For this review, take the finished solid that the model builds, in its own axes (mm). Give positions to 0.01 mm unless a question says otherwise; leave off trailing zeros. Write each loop counter-clockwise with the first axis right and the second up, starting at its lowest first coordinate (ties: lowest second). Pieces come first, ordered by that corner, then holes. Notation, with made-up numbers: (76, 42) -> (92, 42) arc R18 cw to (92, 52) -> close; hole circle Ø7 at (43.25, -0.75). An arc over 180 degrees is marked (long way). Return JSON: item names as keys, results as strings.
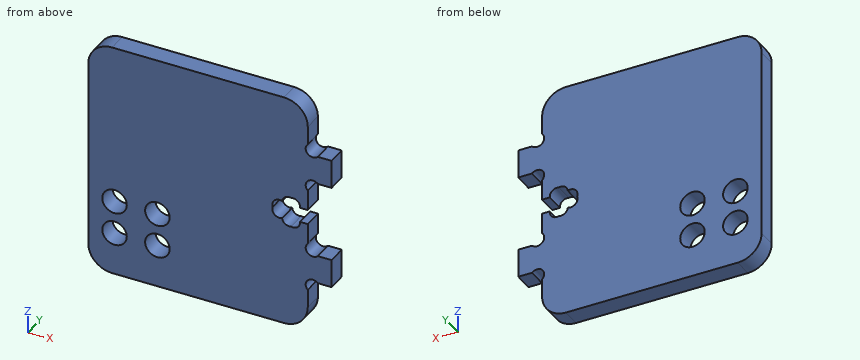
from build123d import *

# Parameters (mm, degrees)
SALIENTE_EXTRUIR1_DEPTH = 4
CORTAR_EXTRUIR4_DEPTH   = 5
CROQUIS10_R             = 1.5
CORTAR_EXTRUIR5_DEPTH   = 5
CROQUIS12_R             = 2.575
CORTAR_EXTRUIR6_DEPTH   = 5


with BuildPart() as part:
    # Croquis1 → Saliente-Extruir1 (new body)
    with BuildSketch(Plane(origin=(0, 0, 0), x_dir=(1, 0, 0), z_dir=(0, 1, 0))):
        with BuildLine():
            Line((-18.025, -25), (18.025, -25))
            ThreePointArc((18.025, -25), (21.560533906, -23.535533906), (23.025, -20))
            Line((23.025, -20), (23.025, -14))
            Line((23.025, -14), (28.025, -14))
            Line((28.025, -14), (28.025, -8))
            Line((28.025, -8), (23.025, -8))
            Line((23.025, -8), (23.025, -1.55))
            Line((23.025, -1.55), (20.975, -1.55))
            Line((20.975, -1.55), (20.975, -2.8))
            Line((20.975, -2.8), (18.075, -2.8))
            Line((18.075, -2.8), (18.075, -1.55))
            Line((18.075, -1.55), (16.025, -1.55))
            Line((16.025, -1.55), (16.025, 1.55))
            Line((16.025, 1.55), (18.075, 1.55))
            Line((18.075, 1.55), (18.075, 2.8))
            Line((18.075, 2.8), (20.975, 2.8))
            Line((20.975, 2.8), (20.975, 1.55))
            Line((20.975, 1.55), (23.025, 1.55))
            Line((23.025, 1.55), (23.025, 8))
            Line((23.025, 8), (28.025, 8))
            Line((28.025, 8), (28.025, 14))
            Line((28.025, 14), (23.025, 14))
            Line((23.025, 14), (23.025, 20))
            ThreePointArc((23.025, 20), (21.560533906, 23.535533906), (18.025, 25))
            Line((18.025, 25), (-18.025, 25))
            ThreePointArc((-18.025, 25), (-21.560533906, 23.535533906), (-23.025, 20))
            Line((-23.025, 20), (-23.025, -20))
            ThreePointArc((-23.025, -20), (-21.560533906, -23.535533906), (-18.025, -25))
        make_face()
    extrude(amount=SALIENTE_EXTRUIR1_DEPTH)

    # Croquis7 → Cortar-Extruir4 (cut, through all)
    with BuildSketch(Plane(origin=(0, 4, 0), x_dir=(1, 0, 0), z_dir=(0, 1, 0))):
        with BuildLine():
            Line((21.402341989, 1.55), (23.025, 1.55))
            Line((23.025, 1.55), (23.025, -1.55))
            Line((23.025, -1.55), (21.402341989, -1.55))
            ThreePointArc((21.402341989, -1.55), (20.900478098, -2.869619136), (19.525, -3.187930349))
            ThreePointArc((19.525, -3.187930349), (18.280747615, -2.971867524), (17.642475162, -1.882163243))
            ThreePointArc((17.642475162, -1.882163243), (16.05076038, -1.575149398), (15.66772275, 0))
            ThreePointArc((15.66772275, 0), (16.05076038, 1.575149398), (17.642475162, 1.882163243))
            ThreePointArc((17.642475162, 1.882163243), (18.280747615, 2.971867524), (19.525, 3.187930349))
            ThreePointArc((19.525, 3.187930349), (20.900478098, 2.869619136), (21.402341989, 1.55))
        make_face()
    extrude(amount=-CORTAR_EXTRUIR4_DEPTH, mode=Mode.SUBTRACT)

    # Croquis10 → Cortar-Extruir5 (cut, through all)
    with BuildSketch(Plane(origin=(0, 4, 0), x_dir=(1, 0, 0), z_dir=(0, 1, 0))):
        with Locations((24.085660172, 15.060660172)):
            Circle(CROQUIS10_R)
        with Locations((24.085660172, 6.939339828)):
            Circle(CROQUIS10_R)
        with Locations((24.085660172, -15.060660172)):
            Circle(CROQUIS10_R)
        with Locations((24.085660172, -6.939339828)):
            Circle(CROQUIS10_R)
    extrude(amount=-CORTAR_EXTRUIR5_DEPTH, mode=Mode.SUBTRACT)

    # Croquis12 → Cortar-Extruir6 (cut, through all)
    with BuildSketch(Plane(origin=(0, 4, 0), x_dir=(1, 0, 0), z_dir=(0, 1, 0))):
        with Locations((-17.525, 16)):
            Circle(CROQUIS12_R)
        with Locations((-8.525, 16)):
            Circle(CROQUIS12_R)
        with Locations((-8.525, 9)):
            Circle(CROQUIS12_R)
        with Locations((-17.525, 9)):
            Circle(CROQUIS12_R)
    extrude(amount=-CORTAR_EXTRUIR6_DEPTH, mode=Mode.SUBTRACT)


solid = part.part
1. To check wall thickness, follow probe 1 along X at (y, z) = (0.35, -16) (3 decimals); probe 2 along Z at (x, y) = (-8, 1.7); probe 3 along Z at (x, y) = (22, 1.6). State the ranges of each line that lie inside material, in increasing order.
Results found:
{"probe 1": "x = -23.025 to -20.1, -14.95 to -11.1, -5.95 to 22.916", "probe 2": "z = -25 to -18.52, -13.48 to -11.52, -6.48 to 25", "probe 3": "z = -23.03 to -1.55, 1.55 to 23.03"}
2. Add section C-C, the plane z = 21.5. State the section outline as (x, y) points.
Results found:
{"outline": "(-22.79, 0) -> (22.79, 0) -> (22.79, 4) -> (-22.79, 4) -> close"}
3. Add section A-A, the plane x = -8.5. State the section outline as (y, z) points, plus the area to 3 significant figures.
Results found:
{"outline": "(0, -25) -> (4, -25) -> (4, -18.57) -> (0, -18.57) -> close; (0, -13.43) -> (4, -13.43) -> (4, -11.57) -> (0, -11.57) -> close; (0, -6.43) -> (4, -6.43) -> (4, 25) -> (0, 25) -> close", "area": "159 mm²"}
4. For pin 1 (1.2 mm diameter, centred on y = 1.5, z = -3.5, fed in from +X) (3 decimals); pin 2 (0.8 mm diameter, centred on x = 22, y = 3, fed in from +Z); pin 3 (0.9 mm diameter, centred on x = 26.5, y = 2, fed in from -Z), all flat-tipped, find the tip position at first contact; note any pin that passes through.
Results found:
{"pin 1": "stops at x = 23.025", "pin 2": "stops at z = 23.5", "pin 3": "stops at z = -14"}
5. Add section B-B, the plane y = 2.15. Count the separate pieces of the cut face and the enclosed holes in it, plus the area to 3 significant figures.
Results found:
{"separate pieces": "1", "enclosed holes": "4", "area": "2,220 mm²"}
